Could you check a few things on this model? Use its own coordinates, in mm. A direction names the side the tool comes from. Give positions to 0.01 mm unless a question says otherwise; leave off trailing zeros. Order: outer loops, then holes, each group sorted by start corner. A loop starts at its lowest first (then second) coordinate and runs counter-clockwise, first axis right, second up. Notation, with made-up numbers: M 89,77 L 101,77 A20 cw 101,88 Z; hole C 9.5,80 d4. An arc over 180 degrees is marked long. Use a Markdown table: item, result. Add a question column.
```python
from build123d import *

# Parameters (mm, degrees)
BOSS_EXTRUDE1_DEPTH = 64.2
CHAMFER1_SIZE       = 0.4
BOSS_EXTRUDE2_DEPTH = 3.4
CHAMFER2_SIZE       = 0.4


with BuildPart() as part:
    # Sketch1 → Boss-Extrude1 (new body)
    with BuildSketch(Plane(origin=(0, 0, 0), x_dir=(1, 0, 0), z_dir=(0, 1, 0))):
        with BuildLine():
            Line((-4.106141741, -6.3), (4.106141741, -6.3))
            ThreePointArc((4.106141741, -6.3), (7.52, 0), (4.106141741, 6.3))
            Line((4.106141741, 6.3), (-4.106141741, 6.3))
            ThreePointArc((-4.106141741, 6.3), (-7.52, 0), (-4.106141741, -6.3))
        make_face()
    extrude(amount=BOSS_EXTRUDE1_DEPTH)

    # Chamfer1
    chamfer1_edges = [part.edges().sort_by_distance(p)[0] for p in [
        (7.52, 64.2, 0),
        (0, 64.2, -6.3),
        (-7.52, 64.2, 0),
        (-7.52, 0, 0),
        (0, 64.2, 6.3),
        (0, 0, -6.3),
        (7.52, 0, 0),
        (0, 0, 6.3),
    ]]
    chamfer(chamfer1_edges, length=CHAMFER1_SIZE)

    # Sketch2 → Boss-Extrude2 (add)
    with BuildSketch(Plane(origin=(0, 40.2, 0), x_dir=(1, 0, 0), z_dir=(0, 1, 0))):
        with BuildLine():
            Line((-7.765951326, -6.3), (7.765951326, -6.3))
            ThreePointArc((7.765951326, -6.3), (10, 0), (7.765951326, 6.3))
            Line((7.765951326, 6.3), (-7.765951326, 6.3))
            ThreePointArc((-7.765951326, 6.3), (-10, 0), (-7.765951326, -6.3))
        make_face()
    extrude(amount=-BOSS_EXTRUDE2_DEPTH)

    # Chamfer2
    chamfer2_edges = [part.edges().sort_by_distance(p)[0] for p in [
        (10, 40.2, 0),
        (-10, 36.8, 0),
        (10, 36.8, 0),
        (-10, 40.2, 0),
    ]]
    chamfer(chamfer2_edges, length=CHAMFER2_SIZE)


solid = part.part
```
1) For pin 1 (5 mm diameter, centred on x = 7.5, y = 33.5, fed in from -Z); pin 2 (6 mm diameter, centred on y = 12, z = -3, fed in from +X); pin 3 (1.6 mm diameter, centred on x = -8, z = -2.5, fed in from +Y), each with a flat end and sliding along its axis, tell me the tip position at first contact or that it passes through.
2) Suppose I cut it at A-A on y = 52.5. Please give me the cut outline in (x, z), and give its area (3 significant figures).
3) Please list where these lines run through material, in increasing order: line 1 (X direction, y = 22, z = -2); line 2 (X direction, y = 3, z = -0.25); line 3 (Y direction, x = -8.5, z = -4). Write a range as from..to.
4) For faces 1 (the face through (8, 40.2, 0)), 2 (the face through (-7.52, 18.35, -0.1)), 3 (the face through (-8, 40.2, 0)), 4 (the face through (8, 36.8, 0)), which set-ups out of +Z, -Z, +X, -X, +Y, -Y let a thin tool reach every point of the face, with its end or its side?
Values found:
| question | item | result |
|---|---|---|
| 1 | pin 1 | stops at z = -5.62 |
| 1 | pin 2 | stops at x = 7.52 |
| 1 | pin 3 | stops at y = 40.2 |
| 2 | outline | M -4.11,-6.3 L 4.11,-6.3 A7.52 ccw 4.11,6.3 L -4.11,6.3 A7.52 ccw Z |
| 2 | area | 164 mm^2 |
| 3 | line 1 | x = -7.25..7.25 |
| 3 | line 2 | x = -7.52..7.52 |
| 3 | line 3 | y = 36.8..40.2 |
| 4 | face 1 | +X, +Y |
| 4 | face 2 | -X, -Y |
| 4 | face 3 | -X, +Y |
| 4 | face 4 | +X, -Y |
